Autodesk Inventor part; units mm, degrees
ref_plane "YZ Plane" through (0, 0, 0) normal (1, 0, 0) x (0, 1, 0)
ref_plane "XZ Plane" through (0, 0, 0) normal (0, 1, 0) x (-1, 0, 0)
ref_plane "XY Plane" through (0, 0, 0) normal (0, 0, 1) x (1, 0, 0)
sketch "Sketch1" plane through (0, 0, 0) normal (0, 0, 1) x (1, 0, 0)
  line L0 (8, 0) -> (67, 0)
  line L1 (67, 0) -> (67, 16)
  line L2 (67, 16) -> (8, 16)
  circle A0 centre (8, 8) radius 1.5
  circle A1 centre (56, 8) radius 6.25
  circle A2 centre (49.75, 8) radius 3.5
  arc A3 (8, 16) -> (8, 0) centre (8, 8) ccw
  point P0 (0, 0)
  point P1 (0, 8)
  point P2 (50.73, 4.64)
  point P3 (50.73, 11.36)
  dimension "d8" = 12.5
  dimension "d0" = 16
  dimension "d2" = 3
  dimension "d3" = 7
  dimension "d4" = 48
  dimension "d6" = 11
  dimension "d7" = 8
  dimension "d9" = 8
  dimension "d10" = 8
extrude "Extrusion1" add sketch "Sketch1" along normal blind 8
sketch "Sketch2" plane through (0, 0, 8) normal (0, 0, 1) x (1, 0, 0)
  line L0 (62.25, 14.25) -> (39.25, 14.25)
  line L1 (39.25, 14.25) -> (39.25, 1.75)
  line L2 (39.25, 1.75) -> (62.25, 1.75)
  line L3 (62.25, 1.75) -> (62.25, 14.25)
  line L4 (67, 16) -> (8, 16)
  line L5 (67, 0) -> (67, 16)
  circle A0 centre (36.75, 8) radius 1
  circle A1 centre (64.75, 8) radius 1
  line L6 (0, 0) -> (67, 0)
  arc A2 (50.73, 4.64) -> (50.73, 11.36) centre (56, 8) ccw
  line L7 (0, 16) -> (0, 0)
  line L8 (0, 0) -> (34.25, 0)
  line L9 (34.25, 0) -> (34.25, 16)
  line L10 (34.25, 16) -> (0, 16)
  line L11 (0, 16) -> (0, 0)
  circle A3 centre (8, 8) radius 1.5
  circle A4 centre (8, 8) radius 2.6
  line L12 (16, 5) -> (34.25, 5)
  line L13 (34.25, 5) -> (34.25, 11)
  line L14 (34.25, 11) -> (16, 11)
  line L15 (16, 11) -> (16, 5)
  dimension "d13" = 23
  dimension "d14" = 12.5
  dimension "d15" = 1.75
  dimension "d19" = 2
  dimension "d20" = 2.5
  dimension "d21" = 2.5
  dimension "d26" = 8
  dimension "d27" = 8
  dimension "d42" = 5
  dimension "d43" = 5.2
  dimension "d44" = 5
  dimension "d45" = 5
  dimension "d53" = 8
extrude "Extrusion2" cut sketch "Sketch2" against normal blind 4 contours L3 A2 L0 | A2 L2 L1 L0 | L3 L2 A2
extrude "Extrusion6" cut sketch "Sketch2" against normal blind 2 contours L9 L14 L15 L12 L6 L7 L10 L4
extrude "Extrusion7" cut sketch "Sketch2" against normal blind 5 contours A4
extrude "Extrusion8" cut sketch "Sketch2" against normal blind 6 contours L9 L12 L15 L14
extrude "Extrusion9" cut sketch "Sketch2" against normal through all contours A0 | A1
properties part number "leg"
The model under review builds one solid part; all positions refer to its coordinate system, in mm. A direction names the side the tool comes from. Coordinates: 2 decimals unless noted, no trailing zeros. Order: outer loops, then holes, each group sorted by start corner. A loop starts at its lowest first (then second) coordinate and runs counter-clockwise, first axis right, second up. Notation, with made-up numbers: (62.5, 27) -> (85.5, 27) arc R25 cw to (85.5, 56) -> close; hole circle Ø6 at (-30.5, 80). An arc over 180 degrees is marked (long way). Answer in a Markdown table with one row per item.
(1) Insertion check: pin 1 (3 mm diameter, centred on x = 53.5, y = 5.5, fed in from +Z); pin 2 (3 mm diameter, centred on y = 4.5, z = 4, fed in from -X); pin 3 (5 mm diameter, centred on x = 29, y = 8, fed in from +Z); pin 4 (6 mm diameter, centred on x = 8, y = 8, fed in from +Z). Each pin has a flat end and moves straight along its axis. Give the tip position at first contact, or say it passes through.
Answers:
| item | result |
|---|---|
| pin 1 | through |
| pin 2 | x = 0.25 |
| pin 3 | z = 2 |
| pin 4 | z = 6 |
(2) The part is to be moulded in two halves that separate along X. For faces 3 (the flat face through (13, 8, 6)), 4 (the cylindrical face through (0, 8, 3)), 5 (the flat face through (25, 8, 2)), say which applies: +X half, -X half, draft (parallel to the pull), parting line (faces both ways), or undercut.
Answers:
| item | result |
|---|---|
| face 3 | draft |
| face 4 | -X half |
| face 5 | undercut |
(3) Consider section A-A (x = 49.75). Write out the cut boundary in (y, z).
Answers:
| item | result |
|---|---|
| outline | (0, 0) -> (4.5, 0) -> (4.5, 4) -> (1.75, 4) -> (1.75, 8) -> (0, 8) -> close; (11.5, 0) -> (16, 0) -> (16, 8) -> (14.25, 8) -> (14.25, 4) -> (11.5, 4) -> close |
(4) Consider section D-D (x = 24). Write out the cut boundary in (y, z).
Answers:
| item | result |
|---|---|
| outline | (0, 0) -> (16, 0) -> (16, 6) -> (11, 6) -> (11, 2) -> (5, 2) -> (5, 6) -> (0, 6) -> close |
(5) Consider section C-C (z = 1). Write out the cut boundary in (x, y), plus the area to 3 significant figures.
Answers:
| item | result |
|---|---|
| outline | (8, 0) -> (67, 0) -> (67, 16) -> (8, 16) arc R8 ccw to start; hole circle Ø3 at (8, 8); hole circle Ø2 at (36.75, 8); hole (50.73, 4.64) arc R6.25 ccw (long way) to (50.73, 11.36) arc R3.5 ccw (long way) to start; hole circle Ø2 at (64.75, 8) |
| area | 887 mm² |
(6) Wall thickness on line 1 along Y through (x, z) = (49.75, 1.65); line 2 along X through (y, z) = (9.25, 1.25); line 3 along Y through (x, z) = (23, 2.25): over which ranges is each line inside the solid? List them lowest first.
Answers:
| item | result |
|---|---|
| line 1 | 0 to 4.5, 11.5 to 16 |
| line 2 | 0.1 to 7.17, 8.83 to 46.48, 62.12 to 67 |
| line 3 | 0 to 5, 11 to 16 |
(7) Consider section B-B (z = 7). Write out the cut boundary in (x, y), plus the area to 3 significant figures.
Answers:
| item | result |
|---|---|
| outline | (34.25, 0) -> (67, 0) -> (67, 16) -> (34.25, 16) -> close; hole circle Ø2 at (36.75, 8); hole (39.25, 1.75) -> (62.25, 1.75) -> (62.25, 14.25) -> (39.25, 14.25) -> close; hole circle Ø2 at (64.75, 8) |
| area | 230 mm² |
(8) Machinability: for faces 1 (the cylindrical face through (63.75, 8.04, 4.06)), 2 (the flat face through (51, 14.25, 6)), which of the approach directions +Z, -Z, +X, -X, +Y, -Y give a long, thin tool a straight path to every point of the face, cutting with its end or side? Answer none if there is none.
Answers:
| item | result |
|---|---|
| face 1 | +Z, -Z |
| face 2 | +Z |
